Can you work these out from the drawing? Everything is in mm from the part's minimum corner. Coordinates: 2 decimals unless noted, no trailing zeros. Write each loop counter-clockwise with the first axis right and the second up, starting at its lowest first coordinate (ties: lowest second). Pieces come first, ordered by that corner, then holes. Notation, with made-up numbers: M -29.5,-25 L -5.5,-25 A20 ccw -5.5,-12 Z; hole C 72.25,86 d9. An arc over 180 degrees is marked long. Write item = value, one per line.
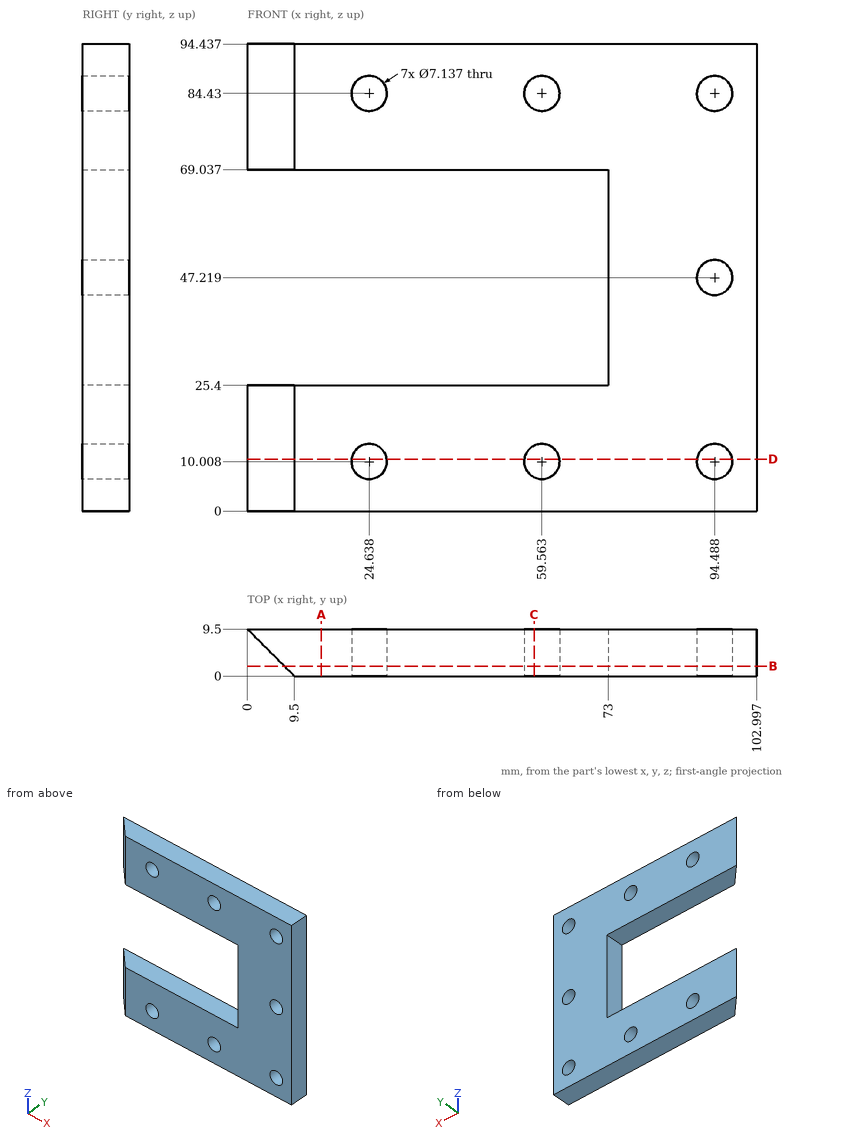
Item 1: Imagine slicing it at B-B (y = 2). Write out the boundary of the cut face in (x, z), and give its area (3 significant figures).
Numbers:
outline = M 7.5,0 L 103,0 L 103,94.44 L 7.5,94.44 L 7.5,69.04 L 73,69.04 L 73,25.4 L 7.5,25.4 Z; hole C 24.64,10.01 d7.14; hole C 24.64,84.43 d7.14; hole C 59.56,10.01 d7.14; hole C 59.56,84.43 d7.14; hole C 94.49,10.01 d7.14; hole C 94.49,47.22 d7.14; hole C 94.49,84.43 d7.14
area = 5,880 mm²
Item 2: Imagine slicing it at C-C (x = 58). Write out the boundary of the cut face in (y, z).
Numbers:
outline = M 0,0 L 9.5,0 L 9.5,6.8 L 0,6.8 Z; M 0,13.22 L 9.5,13.22 L 9.5,25.4 L 0,25.4 Z; M 0,69.04 L 9.5,69.04 L 9.5,81.22 L 0,81.22 Z; M 0,87.64 L 9.5,87.64 L 9.5,94.44 L 0,94.44 Z
Item 3: If I drill on line 1 along Z through (x, y) = (37, 0.75); line 2 along Z through (x, y) = (24, 3); line 3 along X through (y, z) = (1.75, 32), over which ranges is the centre line in solid material (lowest first)?
Numbers:
line_1 = 0 to 25.4, 69.04 to 94.44
line_2 = 0 to 6.5, 13.52 to 25.4, 69.04 to 80.92, 87.94 to 94.44
line_3 = 73 to 103
Item 4: Imagine slicing it at A-A (x = 15). Write out the boundary of the cut face in (y, z).
Numbers:
outline = M 0,0 L 9.5,0 L 9.5,25.4 L 0,25.4 Z; M 0,69.04 L 9.5,69.04 L 9.5,94.44 L 0,94.44 Z
Item 5: Imagine slicing it at D-D (z = 10.5). Write out the boundary of the cut face in (x, y), and give its area (3 significant figures).
Numbers:
outline = M 0,9.5 L 9.5,0 L 21.1,0 L 21.1,9.5 Z; M 28.17,0 L 56.03,0 L 56.03,9.5 L 28.17,9.5 Z; M 63.1,0 L 90.95,0 L 90.95,9.5 L 63.1,9.5 Z; M 98.02,0 L 103,0 L 103,9.5 L 98.02,9.5 Z
area = 732 mm²
Item 6: I'm going to push flat-ended pins straight in: P1, Ø9.5, axis at x = 94.49, z = 84.43, coming from the +Y side; P2, Ø3, axis at y = 7, z = 70, coming from the -X side. Where does each tip first touch, or does it pass through?
Numbers:
P1 = 9.5
P2 = 1
